Geometry check sheet. Reference: the model listing, model coordinates, mm. A direction names the side the tool comes from. Give positions to 0.01 mm unless a question says otherwise; leave off trailing zeros. Loops run counter-clockwise (first coordinate to the right, second up) from the corner with the lowest first, then second, coordinate; pieces in that order, holes last.
1. Cross-section at B-B, the plane y = 0. Record the cut outline in (x, z), plus the area to 3 significant figures.
2. Cross-section at D-D, the plane x = 3.5. Record the cut outline in (y, z), plus the area to 3 significant figures.
3. Tool access check on faces 1 (the flat face through (10, 0, 0)), 2 (the cylindrical face through (27.5, 0.16, 0.49)). Record the directions out of +Z, -Z, +X, -X, +Y, -Y that give a thin tool (end or side, any length) a straight path to the whole face; none if there is none.
4. Cross-section at A-A, the plane z = -0.4. Record the cut outline in (x, y), plus the area to 3 significant figures.
5. Release check for a two-part mould opening along X. For faces 3 (the cylindrical face through (-0.338, -2.578, -0.014)), 4 (the flat face through (9.9, -7.5, 0.5)), 5 (the cylindrical face through (-3, 0.1, -0.5)), 6 (the cylindrical face through (-7.5, -0.16, 0.49)) record: +X half, -X half, draft (parallel to the pull), parting line (faces both ways), or undercut.
6. Material ranges on L1, parallel to Y at x = 20, z = -0.4; L2, parallel to X at y = 2, z = 0.95; L3, parallel to X at y = 1, z = -0.75, recorded low to high.
7. Cross-section at C-C, the plane x = -0.5. Record the cut outline in (y, z).
8. Go/stop test with a flat-tipped pin: pin 1 Ø4 at (x, y) = (20, 0) entering from -Z. Record where the tip stops, or that it passes through.
Autodesk Inventor part; units mm, degrees
ref_plane "YZ Plane" through (0, 0, 0) normal (1, 0, 0) x (0, 1, 0)
ref_plane "XZ Plane" through (0, 0, 0) normal (0, 1, 0) x (-1, 0, 0)
ref_plane "XY Plane" through (0, 0, 0) normal (0, 0, 1) x (1, 0, 0)
sketch "Sketch1" plane through (0, 0, 0) normal (0, 0, 1) x (1, 0, 0)
  circle A0 centre (0, 0) radius 7.5
  circle A1 centre (20, 0) radius 7.5
  line L0 (0, 7.5) -> (20, 7.5)
  line L1 (0, -7.5) -> (20, -7.5)
  circle A2 centre (0, 0) radius 3
  circle A3 centre (20, 0) radius 3
  circle A4 centre (20, 0) radius 2.6
  circle A5 centre (0, 0) radius 2.6
  dimension "d0" = 20
  dimension "d1" = 15
  dimension "d6" = 5.2
  dimension "d7" = 5.2
  dimension "d10" = 0.4
  dimension "d11" = 0.4
  dimension "d12" = 6
extrude "Extrusion1" add sketch "Sketch1" along normal blind 1 contours A0 | A0 L0 A1 L1 | A1 | A2 | A3
extrude "Extrusion2" add sketch "Sketch1" against normal blind 1 contours A2 | A3
equation "\"d6\" = d7"
equation "\"d11\" = d10"
properties part number "Belt Holder"
Result:
1. outline: (-7.5, 0) - (-3, 0) - (-3, -1) - (-2.6, -1) - (-2.6, 1) - (-7.5, 1) - close; (2.6, -1) - (3, -1) - (3, 0) - (17, 0) - (17, -1) - (17.4, -1) - (17.4, 1) - (2.6, 1) - close; (22.6, -1) - (23, -1) - (23, 0) - (27.5, 0) - (27.5, 1) - (22.6, 1) - close
1. area: 26.2 mm2
2. outline: (-7.5, 0) - (7.5, 0) - (7.5, 1) - (-7.5, 1) - close
2. area: 15.0 mm2
3. face 1: -Z
3. face 2: +Z, -Z, +X
4. outline: circle Ø6 at (0, 0); circle Ø6 at (20, 0); hole circle Ø5.2 at (0, 0); hole circle Ø5.2 at (20, 0)
4. area: 14.1 mm2
5. face 3: undercut
5. face 4: draft
5. face 5: undercut
5. face 6: -X half
6. L1: y = -3 to -2.6, 2.6 to 3
6. L2: x = -7.23 to -1.66, 1.66 to 18.34, 21.66 to 27.23
6. L3: x = -2.83 to -2.4, 2.4 to 2.83, 17.17 to 17.6, 22.4 to 22.83
7. outline: (-7.48, 0) - (-2.96, 0) - (-2.96, -1) - (-2.55, -1) - (-2.55, 1) - (-7.48, 1) - close; (2.55, -1) - (2.96, -1) - (2.96, 0) - (7.48, 0) - (7.48, 1) - (2.55, 1) - close
8. pin 1: passes through
